Read the model definition and answer for the solid it produces. Units are mm, in the model's axes. A direction names the side the tool comes from. Coordinates: 2 decimals unless noted, no trailing zeros. Loops run counter-clockwise (first coordinate to the right, second up) from the corner with the lowest first, then second, coordinate; pieces in that order, holes last.
Q1. Which of the six approach directions +Z, -Z, +X, -X, +Y, -Y give full straight-line access (tool end or side, diameter ignored) to faces 1 (the face through (20.5, 0, -20)), 2 (the face through (-28.438, 0, -20)), 3 (the face through (24, 30, -20))?
Q2. Straight lines are drawn through the part: line 1 (Y direction, x = -26.75, z = -40); line 2 (X direction, y = -22.5, z = -10.5); line 3 (Z direction, x = 6, y = -21.5). For each, find the intervals that lie inside material, in ascending order.
Q3. Section B-B (z = -41.5) is taken. Give the vertices of the cut face in (x, y), then the cut area to 3 significant figures.
Q4. The mould has two halves that part along Z. Classify faces 4 (the face through (24.413, 14.166, -38.14)), 5 (the face through (-1, 1, 0)), 6 (the face through (-1, 1, 10)), 7 (the face through (-20.5, 0, -20)): pulls with the +Z half, pulls with the -Z half, needs draft (parallel to the pull), parting line crosses it, or undercut.
Q5. Flat-ended cylindrical pins translate along their axes: P1, Ø5, axis at x = -11.5, y = 39, coming from the -Z side; P2, Ø18, axis at y = 4.5, z = -28, coming from the +X side; P3, Ø8.5, axis at x = 23, z = -26.5, coming from the +Y side. Find the tip coordinate at first contact, or state that the pin passes through.
Q6. Section A-A (y = 0) is taken. Give the vertices of the cut face in (x, z).
Q7. Section C-C (y = -43.5) is taken. Give the vertices of the cut face in (x, z).
from build123d import *

# Parameters (mm, degrees)
SKETCH2_W           = 100
SKETCH2_H           = 100
BOSS_EXTRUDE1_DEPTH = 10
SKETCH3_R           = 14.2875
BOSS_EXTRUDE2_DEPTH = 7.9375
FILLET1_R           = 5


with BuildPart() as part:
    # Sketch2 → Boss-Extrude1 (new body)
    with BuildSketch(Plane.XY):
        Rectangle(SKETCH2_W, SKETCH2_H)
    extrude(amount=BOSS_EXTRUDE1_DEPTH)

    # Sketch3 → Boss-Extrude2 (add)
    with BuildSketch(Plane(origin=(20.5, 0, 0), x_dir=(0, 0, -1), z_dir=(1, 0, 0))):
        with BuildLine():
            Line((0, 30), (40, 30))
            ThreePointArc((40, 30), (70, 0), (40, -30))
            Line((40, -30), (0, -30))
            Line((0, -30), (0, 30))
        make_face()
        with Locations((40, 0)):
            Circle(SKETCH3_R, mode=Mode.SUBTRACT)
    boss_extrude2 = extrude(amount=BOSS_EXTRUDE2_DEPTH)

    # Mirror1: Boss-Extrude2 across plane
    add(boss_extrude2.mirror(Plane(origin=(0, 0, 0), x_dir=(0, 0, 1), z_dir=(1, 0, 0))))

    # Fillet1
    fillet1_edges = [part.edges().sort_by_distance(p)[0] for p in [
        (-50, 50, 5),
        (50, 50, 5),
        (50, -50, 5),
        (-50, -50, 5),
    ]]
    fillet(fillet1_edges, radius=FILLET1_R)


solid = part.part
Numbers:
1. face 1: -Z, +Y, -Y
1. face 2: -Z, -X, +Y, -Y
1. face 3: -Z, +X, -X, +Y
2. line 1: y = -30 to -14.29, 14.29 to 30
2. line 2: x = -28.44 to -20.5, 20.5 to 28.44
2. line 3: z = 0 to 10
3. outline: (-28.44, -29.96) - (-20.5, -29.96) - (-20.5, -14.21) - (-28.44, -14.21) - close; (-28.44, 14.21) - (-20.5, 14.21) - (-20.5, 29.96) - (-28.44, 29.96) - close; (20.5, -29.96) - (28.44, -29.96) - (28.44, -14.21) - (20.5, -14.21) - close; (20.5, 14.21) - (28.44, 14.21) - (28.44, 29.96) - (20.5, 29.96) - close
3. area: 500 mm2
4. face 4: undercut
4. face 5: pulls with the -Z half
4. face 6: pulls with the +Z half
4. face 7: needs draft
5. P1: stops at z = 0
5. P2: stops at x = 28.44
5. P3: stops at y = 30
6. outline: (-50, 0) - (-28.44, 0) - (-28.44, -25.71) - (-20.5, -25.71) - (-20.5, 0) - (20.5, 0) - (20.5, -25.71) - (28.44, -25.71) - (28.44, 0) - (50, 0) - (50, 10) - (-50, 10) - close; (-28.44, -70) - (-20.5, -70) - (-20.5, -54.29) - (-28.44, -54.29) - close; (20.5, -70) - (28.44, -70) - (28.44, -54.29) - (20.5, -54.29) - close
7. outline: (-50, 0) - (50, 0) - (50, 10) - (-50, 10) - close
